Check sheet for the drawn part. Datum: minimum x, y, z corner. Units: mm. Coordinates: 2 decimals unless noted, no trailing zeros. Loops run counter-clockwise (first coordinate to the right, second up) from the corner with the lowest first, then second, coordinate; pieces in that order, holes last. Notation, with made-up numbers: (70.25, -21.75) - (103.25, -21.75) arc R16 ccw to (103.25, 7.25) - close; hole circle Ø10 at (56, 69.5). An arc over 180 degrees is marked (long way). Answer as CSV lines item,"result". Start each with the question number.
1. Material ranges on line 1 (Y direction, x = 52, z = 3.3); line 2 (X direction, y = 31, z = 1.6) (1 decimal); line 3 (Y direction, x = 75, z = 2.1), recorded low to high. Write a range as [from, to].
2. Cross-section at A-A (x = 98). Enter the section's corners in (y, z), plus the area to 3 significant figures.
3. Cross-section at D-D (z = 2.4). Enter the section's corners in (x, y).
4. Cross-section at B-B (y = 22). Enter the section's corners in (x, z).
5. Cross-section at C-C (x = 75). Enter the section's corners in (y, z).
6. Gauge pin test, flat ends, axial feed: P1, Ø1.5, axis at y = 20, z = 1.5, coming from the -X side; P2, Ø1.5, axis at y = 21, z = 3, coming from the -X side. Record the tip position at first contact, or that the pin passes through.
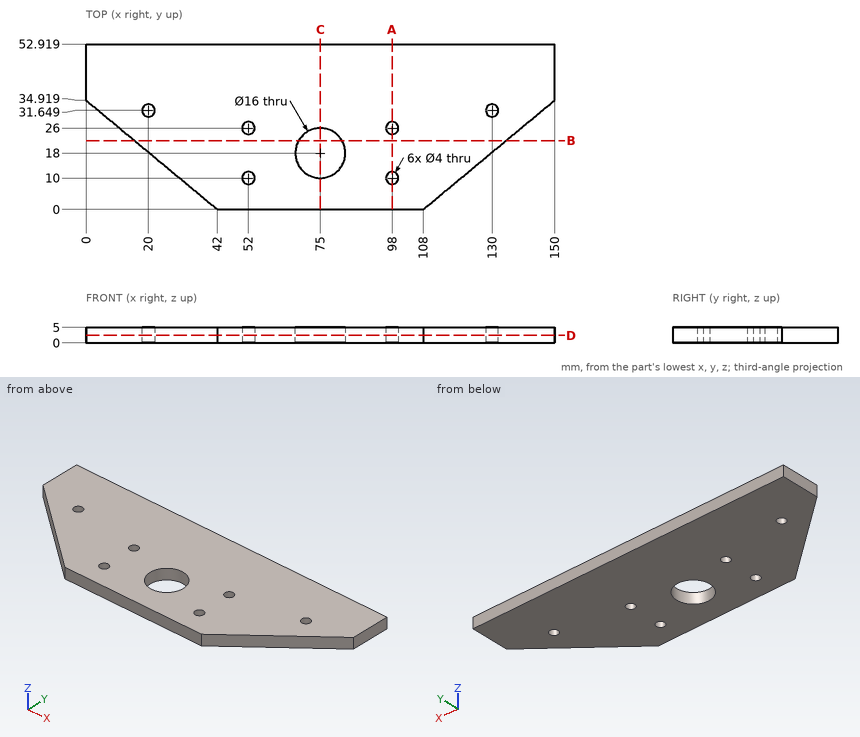
Values follow:
1,line 1,"y = [0, 8], [12, 24], [28, 52.92]"
1,line 2,"x = [4.7, 18.1], [21.9, 128.1], [131.9, 145.3]"
1,line 3,"y = [0, 10], [26, 52.92]"
2,outline,"(0, 0) - (8, 0) - (8, 5) - (0, 5) - close; (12, 0) - (24, 0) - (24, 5) - (12, 5) - close; (28, 0) - (52.92, 0) - (52.92, 5) - (28, 5) - close"
2,area,"225 mm²"
3,outline,"(0, 34.92) - (42, 0) - (108, 0) - (150, 34.92) - (150, 52.92) - (0, 52.92) - close; hole circle Ø4 at (20, 31.65); hole circle Ø4 at (52, 10); hole circle Ø4 at (52, 26); hole circle Ø16 at (75, 18); hole circle Ø4 at (98, 10); hole circle Ø4 at (98, 26); hole circle Ø4 at (130, 31.65)"
4,outline,"(15.54, 0) - (68.07, 0) - (68.07, 5) - (15.54, 5) - close; (81.93, 0) - (134.46, 0) - (134.46, 5) - (81.93, 5) - close"
5,outline,"(0, 0) - (10, 0) - (10, 5) - (0, 5) - close; (26, 0) - (52.92, 0) - (52.92, 5) - (26, 5) - close"
6,P1,"stops at x = 17.04"
6,P2,"stops at x = 15.84"
